Job drawing, mm, ordinate dimensions from the low corner. One solid piece. Give positions to 0.01 mm unless a question says otherwise; leave off trailing zeros. Write each loop counter-clockwise with the first axis right and the second up, starting at its lowest first coordinate (ties: lowest second). Pieces come first, ordered by that corner, then holes. Notation, with made-up numbers: (46, -11) - (92, -11) arc R21 cw to (92, 9) - close; hole circle Ø7 at (45, 77). An arc over 180 degrees is marked (long way). Put each result on its own line as item: value. Start each with the question number.
1. Cut at C-C on x = 2.25. List the corners of the cut face in (y, z).
2. Cut at B-B on y = 0.2. List the corners of the cut face in (x, z) (3 decimals).
3. Drop a flat-ended pin along its axis: pin 1 (1.4 mm diameter, centred on x = 7.75, z = 1.75, fed in from +Y). Give the stop position or say it passes through.
4. Cut at A-A on x = 11.5. List the corners of the cut face in (y, z) (3 decimals).
5. Cut at D-D on x = 9. List the corners of the cut face in (y, z).
6. Wall check: line 1 (X direction, y = 0.1, z = 2.15); line 2 (X direction, y = 0.1, z = 1.85); line 3 (Z direction, x = 7.75, y = 0.25). Give the ranges that are in metal, low to high.
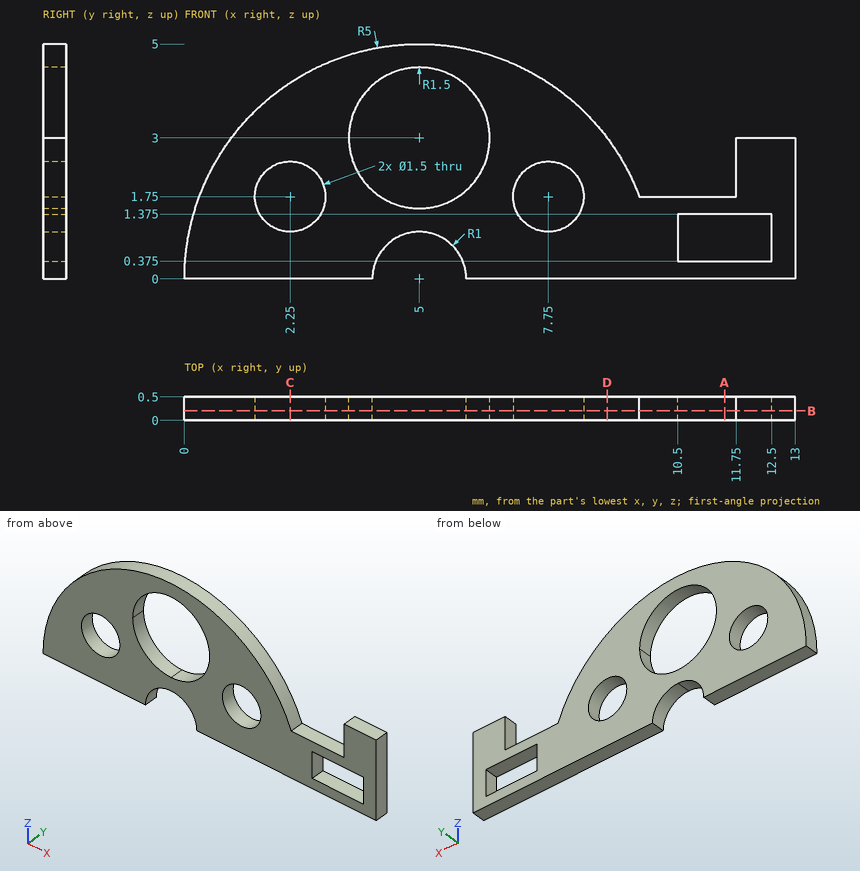
Report:
1. outline: (0, 0) - (0.5, 0) - (0.5, 1) - (0, 1) - close; (0, 2.5) - (0.5, 2.5) - (0.5, 4.18) - (0, 4.18) - close
2. outline: (0, 0) - (4, 0) arc R1 cw to (6, 0) - (13, 0) - (13, 3) - (11.75, 3) - (11.75, 1.75) - (9.684, 1.75) arc R5 ccw to start; hole circle Ø1.5 at (2.25, 1.75); hole circle Ø3 at (5, 3); hole circle Ø1.5 at (7.75, 1.75); hole (10.5, 0.375) - (12.5, 0.375) - (12.5, 1.375) - (10.5, 1.375) - close
3. pin 1: passes through
4. outline: (0, 0) - (0.5, 0) - (0.5, 0.375) - (0, 0.375) - close; (0, 1.375) - (0.5, 1.375) - (0.5, 1.75) - (0, 1.75) - close
5. outline: (0, 0) - (0.5, 0) - (0.5, 3) - (0, 3) - close
6. line 1: x = 0.49 to 1.62, 2.88 to 3.76, 6.24 to 7.12, 8.38 to 9.51, 11.75 to 13
6. line 2: x = 0.35 to 1.51, 2.99 to 4.04, 5.96 to 7.01, 8.49 to 9.65, 11.75 to 13
6. line 3: z = 0 to 1, 2.5 to 4.18
